```python
from build123d import *

# Parameters (mm, degrees)
CYLINDER014005867_R                      = 3.45
CYLINDER014005867_DEPTH                  = 4.1
CYLINDER014005866_R                      = 2.1
CYLINDER014005866_DEPTH                  = 28
FUSION001089102007_PLACEMENT_ANGLE       = 120
FUSION001089102007002_PLACEMENT_ANGLE    = 120
FUSION001089102007003_PLACEMENT_ANGLE    = 180
FUSION001089102007004_PLACEMENT_ANGLE    = 240
FUSION001089102007005_PLACEMENT_ANGLE    = 60
CYLINDER014005868_R                      = 3.15
CYLINDER014005868_DEPTH                  = 28
PRISM002_DEPTH                           = 8.4
CYLINDER014005869_R                      = 2.65
CYLINDER014005869_DEPTH                  = 28
FUSION001089102007007001_PLACEMENT_ANGLE = 180
FUSION001089102007001_PLACEMENT_ANGLE    = 60
CYLINDER014005865_R                      = 35
CYLINDER014005865_DEPTH                  = 12
CYLINDER014005859_R                      = 24.8
CYLINDER014005859_DEPTH                  = 15.9
CHAMFER011_SIZE                          = 0.75


with BuildPart() as obj1:
    # Cylinder014005867 → Cylinder014005867 (new body)
    with BuildSketch(Plane(origin=(0, 23, 24), x_dir=(1, 0, 0), z_dir=(0, 0, 1))):
        Circle(CYLINDER014005867_R)
    extrude(amount=CYLINDER014005867_DEPTH)


with BuildPart() as obj2:
    # Cylinder014005866 → Cylinder014005866 (new body)
    with BuildSketch(Plane(origin=(0, 23, 0), x_dir=(1, 0, 0), z_dir=(0, 0, 1))):
        Circle(CYLINDER014005866_R)
    extrude(amount=CYLINDER014005866_DEPTH)

    # Fusion001089102007: union obj1
    add(obj1.part)


with BuildPart() as obj2_1:
    # Fusion001089102007 placement: moved
    add(obj2.part.rotate(Axis((0, 0, 0), (0, 0, 1)), FUSION001089102007_PLACEMENT_ANGLE))


with BuildPart() as obj3:
    # Fusion001089102007002 base: copy of obj2
    add(obj2_1.part)


with BuildPart() as obj3_1:
    # Fusion001089102007002 placement: moved
    add(obj3.part.rotate(Axis((0, 0, 0), (0, 0, 1)), FUSION001089102007002_PLACEMENT_ANGLE))


with BuildPart() as obj4:
    # Fusion001089102007003 base: copy of obj2
    add(obj2_1.part)


with BuildPart() as obj4_1:
    # Fusion001089102007003 placement: moved
    add(obj4.part.rotate(Axis((0, 0, 0), (0, 0, 1)), FUSION001089102007003_PLACEMENT_ANGLE))


with BuildPart() as obj5:
    # Fusion001089102007004 base: copy of obj2
    add(obj2_1.part)


with BuildPart() as obj5_1:
    # Fusion001089102007004 placement: moved
    add(obj5.part.rotate(Axis((0, 0, 0), (0, 0, 1)), FUSION001089102007004_PLACEMENT_ANGLE))


with BuildPart() as obj6:
    # Fusion001089102007005 base: copy of obj2
    add(obj2_1.part)


with BuildPart() as obj6_1:
    # Fusion001089102007005 placement: moved
    add(obj6.part.rotate(Axis((0, 0, 0), (0, 0, -1)), FUSION001089102007005_PLACEMENT_ANGLE))


with BuildPart() as obj7:
    # Cylinder014005868 → Cylinder014005868 (new body)
    with BuildSketch(Plane.XY):
        Circle(CYLINDER014005868_R)
    extrude(amount=CYLINDER014005868_DEPTH)


with BuildPart() as m4x002:
    # prism002 → prism002 (new body)
    with BuildSketch(Plane(origin=(25, 0, 12), x_dir=(1, 0, 0), z_dir=(0, 0, 1))):
        Polygon((4.6, 0), (2.3, 3.983717), (-2.3, 3.983717), (-4.6, 0), (-2.3, -3.983717), (2.3, -3.983717), align=None)
    extrude(amount=PRISM002_DEPTH)


with BuildPart() as fusion001089102007007:
    # Cylinder014005869 → Cylinder014005869 (new body)
    with BuildSketch(Plane(origin=(25, 0, 12), x_dir=(1, 0, 0), z_dir=(0, 0, 1))):
        Circle(CYLINDER014005869_R)
    extrude(amount=CYLINDER014005869_DEPTH)

    # Fusion001089102007007: union M4X002
    add(m4x002.part)


with BuildPart() as fusion001089102007007001:
    # Fusion001089102007007001 base: copy of Fusion001089102007007
    add(fusion001089102007007.part)


with BuildPart() as fusion001089102007007001_1:
    # Fusion001089102007007001 placement: moved
    add(fusion001089102007007001.part.rotate(Axis((0, 0, 0), (0, 0, 1)), FUSION001089102007007001_PLACEMENT_ANGLE))


with BuildPart() as fusion001089102007006:
    # Fusion001089102007001 base: copy of obj2
    add(obj2_1.part)


with BuildPart() as fusion001089102007006_1:
    # Fusion001089102007001 placement: moved
    add(fusion001089102007006.part.rotate(Axis((0, 0, 0), (0, 0, 1)), FUSION001089102007001_PLACEMENT_ANGLE))

    # Fusion001089102007006: union obj3, obj4, obj5, obj6, obj7, obj2, Fusion001089102007007, Fusion001089102007007001
    add(obj3_1.part)
    add(obj4_1.part)
    add(obj5_1.part)
    add(obj6_1.part)
    add(obj7.part)
    add(obj2_1.part)
    add(fusion001089102007007.part)
    add(fusion001089102007007001_1.part)


with BuildPart() as h005:
    # Cylinder014005865 → Cylinder014005865 (new body)
    with BuildSketch(Plane.XY.offset(15.9)):
        Circle(CYLINDER014005865_R)
    extrude(amount=CYLINDER014005865_DEPTH)


with BuildPart() as obj8:
    # Cylinder014005859 → Cylinder014005859 (new body)
    with BuildSketch(Plane.XY):
        Circle(CYLINDER014005859_R)
    extrude(amount=CYLINDER014005859_DEPTH)

    # Fusion001089102008: union H005
    add(h005.part)

    # Chamfer011
    chamfer011_edges = [obj8.edges().sort_by_distance(p)[0] for p in [
        (-35, 0, 27.9),
        (-35, 0, 15.9),
        (-24.8, 0, 0),
    ]]
    chamfer(chamfer011_edges, length=CHAMFER011_SIZE)

    # Cut009003003009002: cut Fusion001089102007006
    add(fusion001089102007006_1.part, mode=Mode.SUBTRACT)


solid = obj8.part
```
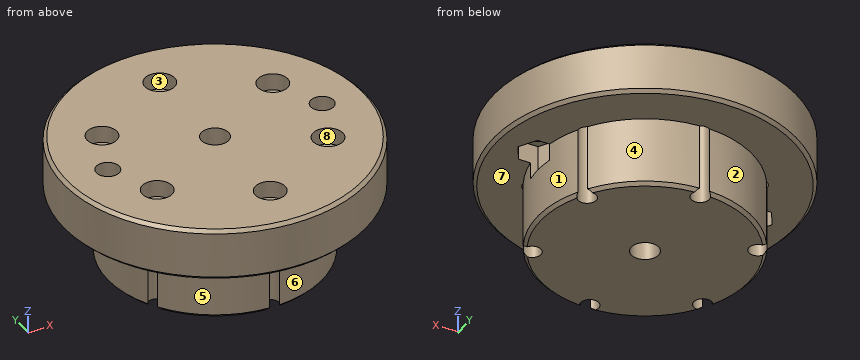
For this review, take the finished solid that the model builds, in its own axes (mm). Face numbers are marked on the shaded views. A direction names the side the tool comes from. Coordinates: 2 decimals unless noted, no trailing zeros. Loops run counter-clockwise (first coordinate to the right, second up) from the corner with the lowest first, then second, coordinate; pieces in that order, holes last. Notation, with made-up numbers: (-1.75, 1.5) -> (49.25, 1.5) arc R21 cw to (49.25, 21.5) -> close; hole circle Ø4 at (-12.5, 47.25). An arc over 180 degrees is marked (long way). Return JSON: item names as keys, results as strings. Group by question number.
(1) Consider section D-D, the plane z = 13. Give the boundary of the cut face in (x, y), plus the area to 3 significant figures.
(2) Consider section B-B, the plane z = 6.25. Give the boundary of the cut face in (x, y), plus the area to 3 significant figures.
(3) Consider section C-C, the plane z = 17.5. Count the separate pieces of the cut face and the enclosed holes in it, plus the area to 3 significant figures.
(4) For pin 1 Ø10 at (x, z) = (15, 18.5) entering from -Y; pin 2 Ø1.4 at (x, z) = (25.5, 15.5) entering from +Y; pin 3 Ø2.5 at (x, z) = (24, 15.5) entering from -Y, all flat-tipped, find the tip position at first contact; note any pin that passes through.
(5) Mouldability with a two-part tool opening along Y and no side actions: class the marked faces 1, 2 and 3 as pulls with the +Y half, pulls with the -Y half, needs draft (parallel to the pull), parting line crosses it, or undercut.
(6) Consider section A-A, the plane x = 0. Give the boundary of the cut face in (y, z).
(7) Tool access review of the marked faces 4, 5, 6, 7 and 8: name each direction out of +Z, -Z, +X, -X, +Y, -Y from which nothing blocks a thin tool from reaching the whole face with its end or side.
(8) To check wall thickness, follow L1, parallel to Y at x = 0, z = 26.55; L2, parallel to X at y = 2, z = 17.25; L3, parallel to X at y = 11.5, z = 16.75. State the ranges of each line that lie inside material, in increasing order.
Results below:
{
 "1": {"outline": "(-24.48, -3.98) arc R24.8 ccw to (-22.02, -11.41) arc R2.1 cw (long way) to (-20.89, -13.36) arc R24.8 ccw to (-1.12, -24.77) arc R2.1 cw (long way) to (1.12, -24.77) arc R24.8 ccw to (20.89, -13.36) arc R2.1 cw (long way) to (22.02, -11.41) arc R24.8 ccw to (24.48, -3.98) -> (22.7, -3.98) -> (20.4, 0) -> (22.7, 3.98) -> (24.48, 3.98) arc R24.8 ccw to (22.02, 11.41) arc R2.1 cw (long way) to (20.89, 13.36) arc R24.8 ccw to (1.12, 24.77) arc R2.1 cw (long way) to (-1.12, 24.77) arc R24.8 ccw to (-20.89, 13.36) arc R2.1 cw (long way) to (-22.02, 11.41) arc R24.8 ccw to (-24.48, 3.98) -> (-22.7, 3.98) -> (-20.4, 0) -> (-22.7, -3.98) -> close; hole circle Ø6.3 at (0, 0)", "area": "1,770 mm2"},
 "2": {"outline": "(-22.02, -11.41) arc R2.1 cw (long way) to (-20.89, -13.36) arc R24.8 ccw to (-1.12, -24.77) arc R2.1 cw (long way) to (1.12, -24.77) arc R24.8 ccw to (20.89, -13.36) arc R2.1 cw (long way) to (22.02, -11.41) arc R24.8 ccw to (22.02, 11.41) arc R2.1 cw (long way) to (20.89, 13.36) arc R24.8 ccw to (1.12, 24.77) arc R2.1 cw (long way) to (-1.12, 24.77) arc R24.8 ccw to (-20.89, 13.36) arc R2.1 cw (long way) to (-22.02, 11.41) arc R24.8 ccw to start; hole circle Ø6.3 at (0, 0)", "area": "1,820 mm2"},
 "3": {"separate pieces": "1", "enclosed holes": "9", "area": "3,620 mm2"},
 "4": {"pin 1": "stops at y = -33.54", "pin 2": "stops at y = 23.56", "pin 3": "stops at y = -25.96"},
 "5": {"face 1": "parting line crosses it", "face 2": "pulls with the +Y half", "face 3": "undercut"},
 "6": {"outline": "(-35, 16.65) -> (-34.25, 15.9) -> (-25.1, 15.9) -> (-25.1, 24) -> (-26.45, 24) -> (-26.45, 27.9) -> (-34.25, 27.9) -> (-35, 27.15) -> close; (-20.9, 0) -> (-3.15, 0) -> (-3.15, 27.9) -> (-19.55, 27.9) -> (-19.55, 24) -> (-20.9, 24) -> close; (3.15, 0) -> (20.9, 0) -> (20.9, 24) -> (19.55, 24) -> (19.55, 27.9) -> (3.15, 27.9) -> close; (25.1, 15.9) -> (34.25, 15.9) -> (35, 16.65) -> (35, 27.15) -> (34.25, 27.9) -> (26.45, 27.9) -> (26.45, 24) -> (25.1, 24) -> close"},
 "7": {"face 4": "-Z, +X, +Y", "face 5": "-Z, -X, -Y", "face 6": "-Z, +X, -Y", "face 7": "-Z", "face 8": "+Z"},
 "8": {"L1": "y = -35 to -26.45, -19.55 to -3.15, 3.15 to 19.55, 26.45 to 35", "L2": "x = -34.94 to -28.45, -21.55 to -2.43, 2.43 to 21.55, 28.45 to 34.94", "L3": "x = -33.06 to -22.02, -17.82 to 17.82, 22.02 to 33.06"}
}
